The listing builds one solid part. Answer for the finished solid, in the listing's coordinates (mm). Coordinates: 2 decimals unless noted, no trailing zeros. Loops run counter-clockwise (first coordinate to the right, second up) from the corner with the lowest first, then second, coordinate; pieces in that order, holes last. Notation, with made-up numbers: (0.25, -10) -> (18.25, -10) arc R37 ccw to (18.25, 29) -> close; hole circle Ø5 at (45.25, -0.5). An arc over 180 degrees is marked (long way). Answer in a Markdown table with one row per item.
```python
from build123d import *

# Parameters (mm, degrees)
SKETCH070_R     = 2.5
PAD030_DEPTH    = 60
SKETCH066_W     = 4
SKETCH066_H     = 4
POCKET022_DEPTH = 16
CHAMFER016_SIZE = 0.3


with BuildPart() as part:
    # Sketch070 → Pad030 (new body)
    with BuildSketch(Plane.XY):
        Circle(SKETCH070_R)
    extrude(amount=PAD030_DEPTH)

    # Sketch066 (on Face3 of Pad030) → Pocket022 (cut)
    with BuildSketch(Plane.XY.offset(60)):
        with Locations((4, 0)):
            Rectangle(SKETCH066_W, SKETCH066_H)
    extrude(amount=-POCKET022_DEPTH, mode=Mode.SUBTRACT)

    # Chamfer016
    chamfer016_edges = [part.edges().sort_by_distance(p)[0] for p in [
        (2.371708, -0.790569, 44),
        (-2.5, 0, 60),
        (2, 0, 60),
    ]]
    chamfer(chamfer016_edges, length=CHAMFER016_SIZE)


with BuildPart() as part_1:
    # Body019 placement: moved
    add(part.part.moved(Location((0, 0, 2))))


solid = part_1.part
```
Item 1: Find the intervals of material crossed by probe 1 along Y at (x, z) = (2, 12); probe 2 along X at (y, z) = (0, 49); probe 3 along Y at (x, z) = (-1.75, 21), in increasing order.
Findings below:
| item | result |
|---|---|
| probe 1 | y = -1.5 to 1.5 |
| probe 2 | x = -2.5 to 2 |
| probe 3 | y = -1.79 to 1.79 |
Item 2: Flat-ended cylindrical pins translate along their axes: pin 1 Ø1 at (x, z) = (1, 24) entering from -Y; pin 2 Ø1.5 at (y, z) = (-1.5, 50.5) entering from +X; pin 3 Ø2 at (x, z) = (-0.5, 15.5) entering from -Y; pin 4 Ø1 at (x, z) = (1.5, 33.5) entering from -Y. Find the tip coordinate at first contact, or state that the pin passes through.
Findings below:
| item | result |
|---|---|
| pin 1 | stops at y = -2.45 |
| pin 2 | stops at x = 2 |
| pin 3 | stops at y = -2.5 |
| pin 4 | stops at y = -2.29 |
Item 3: A cutting plane is placed at B-B, the plane z = 53. Determine the outline of the cut face in (x, y), plus the area to 3 significant figures.
Findings below:
| item | result |
|---|---|
| outline | (2, -1.5) -> (2, 1.5) arc R2.5 ccw (long way) to start |
| area | 18.6 mm2 |
Item 4: A cutting plane is placed at A-A, the plane y = 0. Determine the outline of the cut face in (x, z), plus the area to 3 significant figures.
Findings below:
| item | result |
|---|---|
| outline | (-2.5, 2) -> (2.5, 2) -> (2.5, 45.7) -> (2.2, 46) -> (2, 46) -> (2, 61.7) -> (1.7, 62) -> (-2.2, 62) -> (-2.5, 61.7) -> close |
| area | 292 mm2 |
Item 5: A cutting plane is placed at C-C, the plane z = 22. Determine the outline of the cut face in (x, y), plus the area to 3 significant figures.
Findings below:
| item | result |
|---|---|
| outline | circle Ø5 at (0, 0) |
| area | 19.6 mm2 |
